Read the model definition and answer for the solid it produces. Units are mm, in the model's axes. Face numbers are marked on the shaded views. A direction names the side the tool comes from. Coordinates: 2 decimals unless noted, no trailing zeros. Loops run counter-clockwise (first coordinate to the right, second up) from the corner with the lowest first, then second, coordinate; pieces in that order, holes last. Notation, with made-up numbers: (36, -26.5) -> (62, -26.5) arc R37 ccw to (62, 11.5) -> close; hole circle Ø7 at (79, 73.25). An arc over 180 degrees is marked (long way). Answer as a JSON object with one key per item and string values. Group by question number.
1) Which of the six approach directions +Z, -Z, +X, -X, +Y, -Y give full straight-line access (tool end or side, diameter ignored) to the marked faces 1, 2 and 3?
2) Section D-D, the plane z = 29 is taken. Give the vertices of the cut face in (x, y), plus the area to 3 significant figures.
3) Section C-C, the plane z = 34.5 is taken. Give the vertices of the cut face in (x, y), plus the area to 3 significant figures.
4) Flat-ended cylindrical pins translate along their axes: P1, Ø1.9, axis at x = -1.5, y = -9, coming from the -Z side; P2, Ø1.9, axis at x = 12.02, y = 12.02, coming from the -Z side; P3, Ø4, axis at y = 0.5, z = 6.5, coming from the -X side; P4, Ø4.5, axis at x = 11, y = 12.5, coming from the +Z side. Find the tip coordinate at first contact, or state that the pin passes through.
5) Section A-A, the plane x = 0 is taken. Give the vertices of the cut face in (y, z), plus the area to 3 significant figures.
6) Determine the mould class of the marked faces 4, 5 and 6 for opening direction X: released by +X, released by -X, zero draft, split by the parting line, or undercut.
7) Consider probe 1 along Z at (x, y) = (10, 14); probe 2 along Z at (x, y) = (-6, 9.5); probe 3 along Y at (x, z) = (7, 17.5). Determine where each line is inside the solid, lowest interval first. Write a range as [from, to].
from build123d import *

# Parameters (mm, degrees)
SKETCH1_R             = 13.75
BOSS_EXTRUDE1_DEPTH   = 28
SKETCH2_R             = 8.5
BOSS_EXTRUDE2_DEPTH   = 4
BOSS_EXTRUDE3_DEPTH   = 3
SKETCH5_R             = 1.55
CUT_EXTRUDE1_DEPTH    = 3
BODY_MOVE_COPY1_ANGLE = 45
SKETCH6_R             = 2.5
BOSS_EXTRUDE4_DEPTH   = 18.5


with BuildPart() as part:
    # Sketch1 → Boss-Extrude1 (new body)
    with BuildSketch(Plane.XY):
        Circle(SKETCH1_R)
    extrude(amount=BOSS_EXTRUDE1_DEPTH)

    # Sketch2 → Boss-Extrude2 (add)
    with BuildSketch(Plane.XY.offset(28)):
        Circle(SKETCH2_R)
    extrude(amount=BOSS_EXTRUDE2_DEPTH)

    # Sketch4 → Boss-Extrude3 (add)
    with BuildSketch(Plane(origin=(0, 0, 0), x_dir=(-1, 0, 0), z_dir=(0, 0, -1))):
        with BuildLine():
            Line((-3.5, -17.000000602), (-3.5, -9.5))
            ThreePointArc((-3.5, -9.5), (-5.257359313, -5.257359313), (-9.5, -3.5))
            Line((-9.5, -3.5), (-17, -3.5))
            ThreePointArc((-17, -3.5), (-20.5, 0), (-17, 3.5))
            Line((-17, 3.5), (-9.5, 3.5))
            ThreePointArc((-9.5, 3.5), (-5.257359313, 5.257359313), (-3.5, 9.5))
            Line((-3.5, 9.5), (-3.5, 17.000000602))
            ThreePointArc((-3.5, 17.000000602), (0, 20.5), (3.5, 17.000000602))
            Line((3.5, 17.000000602), (3.5, 9.5))
            ThreePointArc((3.5, 9.5), (5.257359313, 5.257359313), (9.5, 3.5))
            Line((9.5, 3.5), (17, 3.5))
            ThreePointArc((17, 3.5), (20.5, 0), (17, -3.5))
            Line((17, -3.5), (9.5, -3.5))
            ThreePointArc((9.5, -3.5), (5.257359313, -5.257359313), (3.5, -9.5))
            Line((3.5, -9.5), (3.5, -17.000000602))
            ThreePointArc((3.5, -17.000000602), (0, -20.5), (-3.5, -17.000000602))
        make_face()
    extrude(amount=BOSS_EXTRUDE3_DEPTH)

    # Sketch5 → Cut-Extrude1 (cut)
    with BuildSketch(Plane(origin=(0, 0, -3), x_dir=(-1, 0, 0), z_dir=(0, 0, -1))):
        with Locations((0, 17)):
            Circle(SKETCH5_R)
        with Locations((17, 0)):
            Circle(SKETCH5_R)
        with Locations((0, -17)):
            Circle(SKETCH5_R)
        with Locations((-17, 0)):
            Circle(SKETCH5_R)
    extrude(amount=-CUT_EXTRUDE1_DEPTH, mode=Mode.SUBTRACT)


with BuildPart() as part_1:
    # Body-Move/Copy1: moved
    add(part.part.rotate(Axis((0, 0, 0), (0, 0, 1)), BODY_MOVE_COPY1_ANGLE))

    # Sketch6 → Boss-Extrude4 (add)
    with BuildSketch(Plane.XY.offset(32)):
        Circle(SKETCH6_R)
    extrude(amount=BOSS_EXTRUDE4_DEPTH)


solid = part_1.part
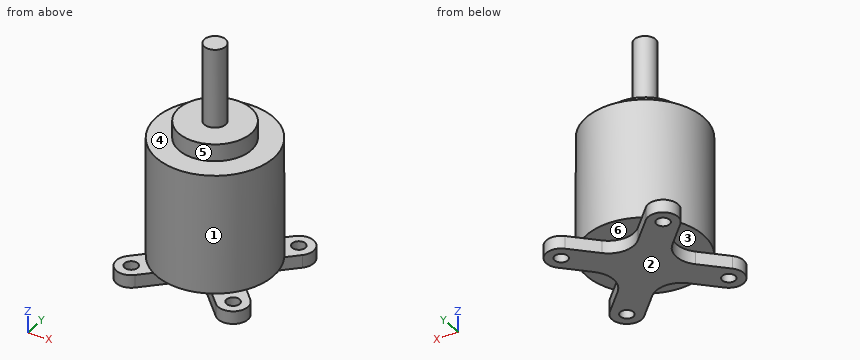
Determined:
{
 "1": {"face 1": "+Z", "face 2": "-Z, +X, -X, +Y, -Y", "face 3": "-Z, -X"},
 "2": {"outline": "circle Ø17 at (0, 0)", "area": "227 mm²"},
 "3": {"outline": "circle Ø5 at (0, 0)", "area": "19.6 mm²"},
 "4": {"P1": "z = 0", "P2": "through", "P3": "x = -13.75", "P4": "z = 0"},
 "5": {"outline": "(-13.75, 0) -> (-7.44, 0) -> (-7.44, -3) -> (7.44, -3) -> (7.44, 0) -> (13.75, 0) -> (13.75, 28) -> (8.5, 28) -> (8.5, 32) -> (2.5, 32) -> (2.5, 50.5) -> (-2.5, 50.5) -> (-2.5, 32) -> (-8.5, 32) -> (-8.5, 28) -> (-13.75, 28) -> close", "area": "975 mm²"},
 "6": {"face 4": "zero draft", "face 5": "split by the parting line", "face 6": "undercut"},
 "7": {"probe 1": "[-3, 0]", "probe 2": "[-3, 28]", "probe 3": "[-11.83, 11.83]"}
}
